Part model, mm, in its own coordinate system. Face numbers are marked on the shaded views. A direction names the side the tool comes from. Give positions to 0.01 mm unless a question says otherwise; leave off trailing zeros. Order: outer loops, then holes, each group sorted by start corner. A loop starts at its lowest first (then second) coordinate and runs counter-clockwise, first axis right, second up. Notation, with made-up numbers: M -27,-24.5 L 12,-24.5 A14 cw 12,0.5 Z; hole C 17,-6.75 d9. An arc over 180 degrees is marked long. Answer as a JSON object with one key per item and string values.
Autodesk Fusion 360 part; units mm, degrees
sketch "Sketch2" plane through (5, 0, 0) normal (1, 0, 0) x (0, 1, 0)
  line L0 (16.9637, 18.2844) -> (-13.0292, -11.7227) construction
  line L1 (-12.9363, 18.2856) -> (17.0619, -11.7162) construction
  circle A0 centre (13.5169, 14.8306) radius 1.6
  circle A1 centre (-9.4831, 14.8306) radius 1.6
  circle A2 centre (-9.4831, -8.1694) radius 1.6
  circle A3 centre (13.5169, -8.1694) radius 1.6
  circle A4 centre (-9.4831, 14.8306) radius 4.1
  circle A5 centre (13.5169, 14.8306) radius 4.1
  circle A6 centre (-9.4831, -8.1694) radius 4.1
  line L2 (9.4619, 10.7862) -> (-5.5274, -4.2245) construction
  line L3 (-7.1431, 18.1972) -> (2.0169, 11.8306)
  line L4 (2.0169, 11.8306) -> (11.1769, 18.1972)
  line L5 (-12.8477, 12.4876) -> (-6.471, 3.3306)
  line L6 (-6.471, 3.3306) -> (-12.8477, -5.8265)
  line L7 (-7.1431, -11.5361) -> (2.0169, -5.1694)
  line L8 (10.5048, 3.3306) -> (16.8815, 12.4876)
  circle A7 centre (13.5169, -8.1694) radius 4.1
  line L9 (10.5048, 3.3306) -> (16.8815, -5.8265)
  line L10 (2.0169, -5.1694) -> (11.1769, -11.5361)
  line L11 (-4.2331, -2.9194) -> (8.2669, -2.9194)
  line L12 (8.2669, -2.9194) -> (8.2669, 9.5806)
  line L13 (8.2669, 9.5806) -> (-4.2331, 9.5806)
  line L14 (-4.2331, 9.5806) -> (-4.2331, -2.9194)
  line L15 (-4.2331, -2.9194) -> (8.2669, 9.5806) construction
  line L16 (8.2669, -2.9194) -> (-4.2331, 9.5806) construction
  line L17 (10.5048, 11.8306) -> (-6.471, 11.8306)
  line L18 (-6.471, 11.8306) -> (-6.471, -5.1694)
  line L19 (-6.471, -5.1694) -> (10.5048, -5.1694)
  line L20 (10.5048, -5.1694) -> (10.5048, 11.8306)
  line L21 (10.5048, 11.8306) -> (-6.471, -5.1694) construction
  line L22 (-6.471, 11.8306) -> (10.5048, -5.1694) construction
  point P0 (2.0169, 3.3306)
  point P1 (2.0169, 3.3306)
  point P2 (2.0169, 3.3306)
  point P3 (2.0169, 3.3306)
  point P4 (2.0169, 3.3306)
  dimension "d11" = 3.2
  dimension "d12" = 11.5
  dimension "d13" = 3.2
  dimension "d14" = 3.2
  dimension "d15" = 3.2
  dimension "d18" = 11.5
  dimension "d19" = 23
  dimension "d20" = 8.2
  dimension "d21" = 8.2
  dimension "d22" = 8.2
  dimension "d23" = 8.2
  dimension "d33" = 12.5
  dimension "d34" = 17
  dimension "d35" = 23
extrude "Extrude12" add sketch "Sketch2" along normal blind 5
extrude "Extrude13" add sketch "Sketch2" against normal blind 5 contours L17 L18 L19 L20
extrude "Extrude3" [suppressed]
equation "d11 = motorScrewHole"
equation "d12 = boltDistance / 2"
equation "d13 = motorScrewHole"
equation "d14 = motorScrewHole"
equation "d15 = motorScrewHole"
equation "motorScrewHole = 3.2 mm"
equation "d18 = boltDistance / 2"
equation "d19 = boltDistance"
equation "d20 = motorScrewHole + 5 mm"
equation "d21 = motorScrewHole + 5 mm"
equation "d22 = motorScrewHole + 5 mm"
equation "d23 = motorScrewHole + 5 mm"
equation "d35 = boltDistance"
equation "boltDistance = 23 mm"
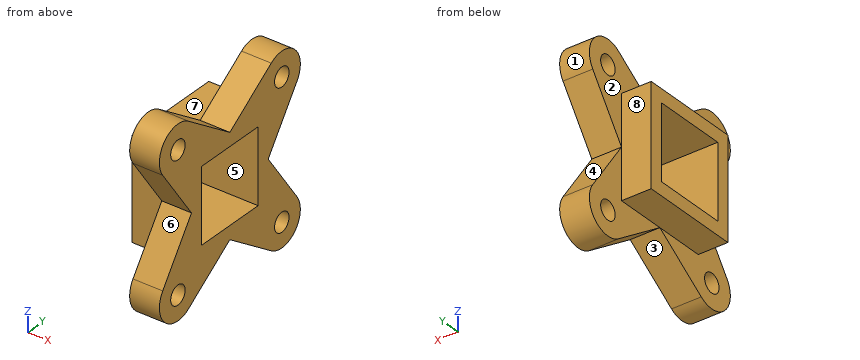
1. Probe line 1 along Z through (x, y) = (3.75, 4.5); line 2 along Y through (x, z) = (1.75, 6); line 3 along Z through (x, y) = (7.75, 14). List the from-to ranges inside material, lowest first.
Worked answers:
{"line 1": "z = -5.17 to -2.92, 9.58 to 11.83", "line 2": "y = -6.47 to -4.23, 8.27 to 10.5", "line 3": "z = -12.24 to -9.69, -6.64 to -1.69, 8.35 to 13.31, 16.36 to 18.9"}
2. Which spindle directions (+Z, -Z, +X, -X, +Y, -Y) get a long thin tool onto all of the face, cutting with end or side? Do the marked faces 4, 5, 6, 7 and 8. Say none if no direction does.
Worked answers:
{"face 4": "+X, -X, +Y", "face 5": "+X, -X", "face 6": "+X, -X, -Y", "face 7": "+Z, -X, +Y, -Y", "face 8": "+Z, -Z, -X, +Y"}
3. Cut at C-C on z = 0. Give the cut face in (x, y).
Worked answers:
{"outline": "M 0,-6.47 L 5,-6.47 L 5,-8.79 L 10,-8.79 L 10,-4.23 L 0,-4.23 Z; M 0,8.27 L 10,8.27 L 10,12.82 L 5,12.82 L 5,10.5 L 0,10.5 Z"}
4. Cut at A-A on y = 0. Give the cut face in (x, z).
Worked answers:
{"outline": "M 0,-5.17 L 5,-5.17 L 5,-6.57 L 10,-6.57 L 10,-2.92 L 0,-2.92 Z; M 0,9.58 L 10,9.58 L 10,13.23 L 5,13.23 L 5,11.83 L 0,11.83 Z"}
5. Two-plate mould, pull along Z, no slides. Class the marked faces 1, 2 and 3: +Z half, -Z half, draft (parallel to the pull), parting line (faces both ways), or undercut.
Worked answers:
{"face 1": "undercut", "face 2": "draft", "face 3": "-Z half"}
6. Cut at B-B on x = 1.25. Give the cut face in (y, z), plus the area to 3 significant figures.
Worked answers:
{"outline": "M -6.47,-5.17 L 10.5,-5.17 L 10.5,11.83 L -6.47,11.83 Z; hole M -4.23,-2.92 L 8.27,-2.92 L 8.27,9.58 L -4.23,9.58 Z", "area": "132 mm^2"}
7. Cut at D-D on x = 8.5. Give the cut face in (y, z), plus the area to 3 significant figures.
Worked answers:
{"outline": "M -12.85,-5.83 A4.1 ccw -7.14,-11.54 L 2.02,-5.17 L 11.18,-11.54 A4.1 ccw 16.88,-5.83 L 10.5,3.33 L 16.88,12.49 A4.1 ccw 11.18,18.2 L 2.02,11.83 L -7.14,18.2 A4.1 ccw -12.85,12.49 L -6.47,3.33 Z; hole C -9.48,-8.17 d3.2; hole C -9.48,14.83 d3.2; hole M -4.23,-2.92 L 8.27,-2.92 L 8.27,9.58 L -4.23,9.58 Z; hole C 13.52,-8.17 d3.2; hole C 13.52,14.83 d3.2", "area": "479 mm^2"}
8. Pin check, flat tips, straight feed: P1, Ø3.5, axis at y = 13.52, z = 14.83, coming from the -X side; P2, Ø4, axis at x = 9, z = -4, coming from the +Y side; P3, Ø1.5, axis at x = 1.5, y = -1.5, coming from the -Z side. Stop position of each tip, or through.
Worked answers:
{"P1": "stops at x = 5", "P2": "stops at y = 17", "P3": "stops at z = -5.17"}
